Autodesk Inventor part; units mm, degrees
ref_plane "YZ Plane" through (0, 0, 0) normal (1, 0, 0) x (0, 1, 0)
ref_plane "XZ Plane" through (0, 0, 0) normal (0, 1, 0) x (-1, 0, 0)
ref_plane "XY Plane" through (0, 0, 0) normal (0, 0, 1) x (1, 0, 0)
sketch "Sketch1" plane through (0, 0, 0) normal (0, 0, 1) x (1, 0, 0)
  line L0 (55, -50) -> (-55, -50)
  line L1 (-55, -50) -> (-55, 50)
  line L2 (-55, 50) -> (55, 50)
  line L3 (55, 50) -> (55, -50)
  line L4 (55, -50) -> (-55, 50) construction
  line L5 (-55, -50) -> (55, 50) construction
  point P0 (0, 0)
  dimension "d0" = 110
  dimension "d1" = 100
extrude "Extrusion1" add sketch "Sketch1" along normal blind 10
sketch "Sketch2" plane through (0, 0, 10) normal (0, 0, 1) x (1, 0, 0)
  line L0 (53, -48) -> (-53, -48)
  line L1 (-53, -48) -> (-53, 48)
  line L2 (-53, 48) -> (53, 48)
  line L3 (53, 48) -> (53, -48)
  line L4 (53, -48) -> (-53, 48) construction
  line L5 (-53, -48) -> (53, 48) construction
  point P0 (0, 0)
  dimension "d4" = 106
  dimension "d5" = 96
extrude "Extrusion2" cut sketch "Sketch2" against normal blind 8
fillet "Fillet1" radius 10 4 edges at (-55, -50, 5) (-53, -48, 6) (55, -50, 5) (53, -48, 6)
sketch "Sketch3" plane through (-55, 50, 0) normal (-1, 0, 0) x (0, 0, 1)
  line L0 (0, 0) -> (10, 0)
  line L1 (10, 0) -> (16, 0)
  line L2 (16, 0) -> (16, -50)
  line L3 (16, -50) -> (14, -50)
  line L4 (14, -50) -> (14, -2)
  line L5 (14, -2) -> (10, -2)
  line L6 (10, -90) -> (10, 0)
  point P0 (0, -50)
  dimension "d9" = 50
  dimension "d10" = 6
  dimension "d11" = 4
  dimension "d12" = 2
extrude "Extrusion3" add sketch "Sketch3" against normal blind 2
sketch "Sketch4" plane through (55, 50, 10) normal (1, 0, 0) x (0, 0, -1)
  line L0 (10, 0) -> (0, 0)
  line L1 (10, 0) -> (-6, 0)
  line L2 (0, 0) -> (-6, 0)
  line L3 (-6, 0) -> (-6, -50)
  line L4 (-6, 0) -> (-6, -50)
  line L5 (-6, -50) -> (-4, -50)
  line L6 (-6, -50) -> (-4, -50)
  line L7 (-4, -50) -> (-4, -2)
  line L8 (-4, -50) -> (-4, -2)
  line L9 (-4, -2) -> (0, -2)
  line L10 (0, -90) -> (0, 0)
  point P0 (10, -50)
extrude "Extrusion4" add sketch "Sketch4" against normal blind 2
fillet "Fillet2" radius 10 2 edges at (-54, 0, 16) (54, 0, 16)
fillet "Fillet3" radius 2 8 edges at (-54, 50, 16) (54, 50, 16) (-54, 48, 14) (54, 48, 14) (54, 48, 10) (-54, 48, 10) (-53, 49, 10) (53, 49, 10)
properties part number "backpack"
Build history of the part. All positions in model axes, mm. A direction names the side the tool comes from. Coordinates: 2 decimals unless noted, no trailing zeros. Write each loop counter-clockwise with the first axis right and the second up, starting at its lowest first coordinate (ties: lowest second). Pieces come first, ordered by that corner, then holes.
(1) Cut at B-B on y = 11.5. List the corners of the cut face in (x, z).
(2) Drill centre lines: line 1 (X direction, y = 2, z = 9); line 2 (Y direction, x = 25, z = 8.75); line 3 (Z direction, x = 9, y = -4.5). Where is each one in solid material? Low to high.
(3) Cut at C-C on x = 3.5. List the corners of the cut face in (y, z).
(4) Pin check, flat tips, straight feed: pin 1 Ø12 at (x, y) = (37, -39.5) entering from +Z; pin 2 Ø2 at (x, y) = (-25.5, 49) entering from +Z. Stop position of each tip, or through.
(5) Cut at A-A on z = 5.75. List the corners of the cut face in (x, y).
(6) 3-axis set-ups, long thin cutter, end or side, ignore diameter. For faces 4 (the flat face through (1, 48, 6)), 5 (the flat face through (-1, 1, 0)), 6 (the flat face through (53, 25, 15)): which of +Z, -Z, +X, -X, +Y, -Y reach the whole face in a straight line?
(7) Mould opens along Y. For faces 1 (the flat face through (53, 6, 6)), 2 (the cylindrical face through (51.99, -47.15, 5.07)), 3 (the flat face through (-53.2, -8.9, 10)) say: pulls with the +Y half, pulls with the -Y half, needs draft (parallel to the pull), parting line crosses it, or undercut.
(8) Cut at D-D on y = -14. List the corners of the cut face in (x, z).
Working result:
1. outline: (-55, 0) - (55, 0) - (55, 10) - (53, 10) - (53, 2) - (-53, 2) - (-53, 10) - (-55, 10) - close; (-55, 14) - (-53, 14) - (-53, 16) - (-55, 16) - close; (53, 14) - (55, 14) - (55, 16) - (53, 16) - close
2. line 1: x = -55 to -53, 53 to 55
2. line 2: y = -50 to -48, 48 to 50
2. line 3: z = 0 to 2
3. outline: (-50, 0) - (50, 0) - (50, 10) - (48, 10) - (48, 2) - (-48, 2) - (-48, 10) - (-50, 10) - close
4. pin 1: stops at z = 2
4. pin 2: stops at z = 10
5. outline: (-55, -40) arc R10 ccw to (-45, -50) - (45, -50) arc R10 ccw to (55, -40) - (55, 50) - (-55, 50) - close; hole (-53, -38) arc R10 ccw to (-43, -48) - (43, -48) arc R10 ccw to (53, -38) - (53, 48) - (-53, 48) - close
6. face 4: +Z
6. face 5: -Z, +X, -X, +Y, -Y
6. face 6: +Z, +Y, -Y
7. face 1: undercut
7. face 2: pulls with the -Y half
7. face 3: needs draft
8. outline: (-55, 0) - (55, 0) - (55, 10) - (53, 10) - (53, 2) - (-53, 2) - (-53, 10) - (-55, 10) - close
